from build123d import *

# Parameters (mm, degrees)
SKETCH_1_R          = 12.5
EXTRUDE_1_DEPTH     = 5
SKETCH_2_R          = 1.1
CUT_EXTRUDE_1_DEPTH = 19.371173071
SKETCH_2_3_R        = 2
CUT_EXTRUDE_2_DEPTH = 3
SKETCH_3_W          = 12
SKETCH_3_H          = 5
EXTRUDE_2_DEPTH     = 20
SKETCH_4_R          = 3
CUT_EXTRUDE_3_DEPTH = 32.721443851


with BuildPart() as part:
    # 草图1 → 凸台-拉伸1 (new body)
    with BuildSketch(Plane(origin=(0, 0, 0), x_dir=(1, 0, 0), z_dir=(0, 1, 0))):
        with Locations(Location((0, 0, 0), (0, 0, 270))):
            Circle(SKETCH_1_R)
    extrude(amount=EXTRUDE_1_DEPTH)

    # 草图2 → 切除-拉伸1 (cut, through all)
    with BuildSketch(Plane(origin=(0, 5, 0), x_dir=(1, 0, 0), z_dir=(0, 1, 0))):
        with Locations(Location((0, -9.5, 0), (0, 0, 270))):
            Circle(SKETCH_2_R)
        with Locations(Location((0, 9.5, 0), (0, 0, 270))):
            Circle(SKETCH_2_R)
        with Locations(Location((9.5, 0, 0), (0, 0, 270))):
            Circle(SKETCH_2_R)
        with Locations(Location((-9.5, 0, 0), (0, 0, 270))):
            Circle(SKETCH_2_R)
    extrude(amount=-CUT_EXTRUDE_1_DEPTH, mode=Mode.SUBTRACT)

    # 草图2<3> → 切除-拉伸2 (cut)
    with BuildSketch(Plane(origin=(0, 5, 0), x_dir=(1, 0, 0), z_dir=(0, 1, 0))):
        with Locations(Location((-9.5, 0, 0), (0, 0, 270))):
            Circle(SKETCH_2_3_R)
        with Locations(Location((0, 9.5, 0), (0, 0, 270))):
            Circle(SKETCH_2_3_R)
        with Locations(Location((9.5, 0, 0), (0, 0, 270))):
            Circle(SKETCH_2_3_R)
        with Locations(Location((0, -9.5, 0), (0, 0, 270))):
            Circle(SKETCH_2_3_R)
    extrude(amount=-CUT_EXTRUDE_2_DEPTH, mode=Mode.SUBTRACT)

    # 草图3 → 凸台-拉伸2 (add)
    with BuildSketch(Plane(origin=(0, 5, 0), x_dir=(1, 0, 0), z_dir=(0, 1, 0))):
        Rectangle(SKETCH_3_W, SKETCH_3_H)
    extrude(amount=EXTRUDE_2_DEPTH)

    # 草图4 → 切除-拉伸3 (cut, through all)
    with BuildSketch(Plane(origin=(0, 0, -2.5), x_dir=(-1, 0, 0), z_dir=(0, 0, -1))):
        with BuildLine():
            ThreePointArc((0, 25), (4.242640687, 23.242640687), (6, 19))
            Line((6, 19), (6, 25))
            Line((6, 25), (0, 25))
        make_face()
        with BuildLine():
            ThreePointArc((-6, 19), (-4.242640687, 23.242640687), (0, 25))
            Line((0, 25), (-6, 25))
            Line((-6, 25), (-6, 19))
        make_face()
        with Locations((0, 19)):
            Circle(SKETCH_4_R)
    extrude(amount=-CUT_EXTRUDE_3_DEPTH, mode=Mode.SUBTRACT)


solid = part.part
Part model, mm, in its own coordinate system. A direction names the side the tool comes from. Coordinates: 2 decimals unless noted, no trailing zeros. Order: outer loops, then holes, each group sorted by start corner. A loop starts at its lowest first (then second) coordinate and runs counter-clockwise, first axis right, second up.
(1) Probe L1, parallel to X at y = 0.6, z = 0; L2, parallel to Z at x = 4.75, y = 20.25; L3, parallel to Y at x = -5, z = -5. List the from-to ranges inside material, lowest first.
Check sheet entries:
L1: x = -12.5 to -10.6, -8.4 to 8.4, 10.6 to 12.5
L2: z = -2.5 to 2.5
L3: y = 0 to 5
(2) Tool access for faces 1 (the face through (-6, 12, 0)), 2 (the face through (0, 13, -2.5)), 3 (the face through (-0.9, 2, 10.4)): list every direction of +Z, -Z, +X, -X, +Y, -Y with a clear straight run to the whole face (end or side of a thin tool).
Check sheet entries:
face 1: +Z, -Z, -X, +Y
face 2: -Z, +X, -X, +Y
face 3: +Y
(3) Slice it at C-C, the plane z = 10. Write the cut outline in (x, y).
Check sheet entries:
outline: (-7.5, 0) - (-0.98, 0) - (-0.98, 2) - (-1.94, 2) - (-1.94, 5) - (-7.5, 5) - close; (0.98, 0) - (7.5, 0) - (7.5, 5) - (1.94, 5) - (1.94, 2) - (0.98, 2) - close
(4) Pull direction X, two halves, no side cores. Call faces 4 (the face through (3.755, 2.465, 11.923)), 5 (the face through (6, 12, 0)), 6 (the face through (0.65, 16.07, -0.04)): pulls with the +X half, pulls with the -X half, needs draft (parallel to the pull), parting line crosses it, or undercut.
Check sheet entries:
face 4: parting line crosses it
face 5: pulls with the +X half
face 6: undercut
(5) Pin check, flat tips, straight feed: pin 1 Ø1.3 at (x, z) = (0, 9.5) entering from +Y; pin 2 Ø5 at (x, z) = (9.5, 0) entering from +Y; pin 3 Ø1.5 at (y, z) = (9, 1) entering from -X; pin 4 Ø2.5 at (y, z) = (15, 0.5) entering from +X. Stop position of each tip, or through.
Check sheet entries:
pin 1: passes through
pin 2: stops at y = 5
pin 3: stops at x = -6
pin 4: stops at x = 6
(6) Slice it at D-D, the plane x = -9.5. Write the cut outline in (y, z).
Check sheet entries:
outline: (0, -8.12) - (5, -8.12) - (5, -2) - (2, -2) - (2, -1.1) - (0, -1.1) - close; (0, 1.1) - (2, 1.1) - (2, 2) - (5, 2) - (5, 8.12) - (0, 8.12) - close
(7) Slice it at A-A, the plane z = 0. Write the cut outline in (x, y).
Check sheet entries:
outline: (-12.5, 0) - (-10.6, 0) - (-10.6, 2) - (-11.5, 2) - (-11.5, 5) - (-12.5, 5) - close; (-8.4, 0) - (8.4, 0) - (8.4, 2) - (7.5, 2) - (7.5, 5) - (6, 5) - (6, 19) arc R6 ccw to (-6, 19) - (-6, 5) - (-7.5, 5) - (-7.5, 2) - (-8.4, 2) - close; (10.6, 0) - (12.5, 0) - (12.5, 5) - (11.5, 5) - (11.5, 2) - (10.6, 2) - close; hole circle Ø6 at (0, 19)
(8) Slice it at B-B, the plane y = 3. Write the cut outline in (x, z).
Check sheet entries:
outline: circle Ø25 at (0, 0); hole circle Ø4 at (-9.5, 0); hole circle Ø4 at (0, -9.5); hole circle Ø4 at (0, 9.5); hole circle Ø4 at (9.5, 0)
